from build123d import *

# Parameters (mm, degrees)
F1_W     = 50.8
F1_H     = 50.8
F1_W_2   = 38.1
F1_H_2   = 38.1
F4_DEPTH = 50.801
F6_DEPTH = 50.801


with BuildPart() as f2:
    # F2: sweep along a path in F0
    with BuildLine(Plane.XY) as f2_path:
        Line((0, 0), (0, 584.2))
        Line((0, 584.2), (-584.2, 584.2))
    # F1 (on Front) → F2 (sweep)
    with BuildSketch(Plane.XZ):
        Rectangle(F1_W, F1_H)
        Rectangle(F1_W_2, F1_H_2, mode=Mode.SUBTRACT)
    sweep(path=f2_path.line, transition=Transition.RIGHT)

    # F3 (on face) → F4 (cut, through all)
    with BuildSketch(Plane(origin=(-25.4, 0, 0), x_dir=(0, -1, 0), z_dir=(-1, 0, 0))):
        Polygon((0, -25.4), (0, 25.4), (-50.8, -25.4), align=None)
    extrude(amount=-F4_DEPTH, mode=Mode.SUBTRACT)

    # F5 (on face) → F6 (cut, through all)
    with BuildSketch(Plane.XZ.offset(-558.8)):
        Polygon((-584.2, 25.4), (-584.2, -25.4), (-533.4, -25.4), align=None)
    extrude(amount=-F6_DEPTH, mode=Mode.SUBTRACT)


solid = f2.part
The listing builds one solid part. Answer for the finished solid, in the listing's coordinates (mm). A direction names the side the tool comes from. Coordinates: 2 decimals unless noted, no trailing zeros. Loops run counter-clockwise (first coordinate to the right, second up) from the corner with the lowest first, then second, coordinate; pieces in that order, holes last.
1) Determine the mould class of faces 1 (the face through (22.2, 25, 0.4)), 2 (the face through (-25.4, 283, 0)), 3 (the face through (19.05, 309, 0)) for opening direction X: pulls with the +X half, pulls with the -X half, needs draft (parallel to the pull), parting line crosses it, or undercut.
2) Find section B-B on y = 130.5. Write down the section's boundary in (x, z), then the cut area to 3 significant figures.
3) Find section A-A on z = 2. Write down the section's boundary in (x, y), then the cut area to 3 significant figures.
4) Find section C-C on x = -378. Write down the section's boundary in (y, z).
5) Find the intervals of material crossed by L1, parallel to Y at x = -180.5, z = 3; L2, parallel to X at y = 475.5, z = -18; L3, parallel to X at y = 248.5, z = -22, in increasing order.
6) Flat-ended cylindrical pins translate along their axes: pin 1 Ø3 at (y, z) = (513, 19.5) entering from -X; pin 2 Ø19 at (x, z) = (-160.5, 1) entering from -Y. Find the tip coordinate at first contact, or state that the pin passes through.
7) A tool of negligible diameter and unlimited length cuts with its end or side. For faces 4 (the face through (-19.05, 290, 0)), 5 (the face through (-309, 558.8, 0)), 6 (the face through (-302, 565.15, 0)), 7 (the face through (-11, 449, -19.05)), from which of +Z, -Z, +X, -X, +Y, -Y can it reach the whole face along a straight path? Write none if from no direction.
Values:
1. face 1: needs draft
1. face 2: pulls with the -X half
1. face 3: undercut
2. outline: (-25.4, -25.4) - (25.4, -25.4) - (25.4, 25.4) - (-25.4, 25.4) - close; hole (-19.05, -19.05) - (19.05, -19.05) - (19.05, 19.05) - (-19.05, 19.05) - close
2. area: 1,130 mm2
3. outline: (-560.8, 558.8) - (-25.4, 558.8) - (-25.4, 23.4) - (-19.05, 23.4) - (-19.05, 565.15) - (-560.8, 565.15) - close; (-560.8, 603.25) - (19.05, 603.25) - (19.05, 23.4) - (25.4, 23.4) - (25.4, 609.6) - (-560.8, 609.6) - close
3. area: 14,200 mm2
4. outline: (558.8, -25.4) - (609.6, -25.4) - (609.6, 25.4) - (558.8, 25.4) - close; hole (565.15, -19.05) - (603.25, -19.05) - (603.25, 19.05) - (565.15, 19.05) - close
5. L1: y = 558.8 to 565.15, 603.25 to 609.6
5. L2: x = -25.4 to -19.05, 19.05 to 25.4
5. L3: x = -25.4 to 25.4
6. pin 1: stops at x = -25.4
6. pin 2: stops at y = 558.8
7. face 4: -Y
7. face 5: +Z, -Z, -X, -Y
7. face 6: -X
7. face 7: none
